from build123d import *

# Parameters (mm, degrees)
SKETCH_1_R          = 70
SKETCH_1_R_2        = 68.5
EXTRUDE_1_DEPTH     = 8
SKETCH_2_R          = 68.5
SKETCH_2_R_2        = 64
EXTRUDE_2_DEPTH     = 3
SKETCH_3_R          = 64
SKETCH_3_R_2        = 62.5
EXTRUDE_3_DEPTH     = 100
EXTRUDE_START       = 97
SKETCH_4_R          = 62.5
EXTRUDE_4_DEPTH     = 3
SKETCH_5_W          = 10
SKETCH_5_H          = 10
CUT_EXTRUDE_1_DEPTH = 10


with BuildPart() as part:
    # 스케치1 → 보스-돌출1 (new body)
    with BuildSketch(Plane(origin=(0, 0, 0), x_dir=(1, 0, 0), z_dir=(0, 1, 0))):
        with Locations(Location((0, 0, 0), (0, 0, 270))):
            Circle(SKETCH_1_R)
        with Locations(Location((0, 0, 0), (0, 0, 270))):
            Circle(SKETCH_1_R_2, mode=Mode.SUBTRACT)
    extrude(amount=EXTRUDE_1_DEPTH)

    # 스케치2 → 보스-돌출2 (add)
    with BuildSketch(Plane(origin=(0, 0, 0), x_dir=(1, 0, 0), z_dir=(0, 1, 0))):
        with Locations(Location((0, 0, 0), (0, 0, 270))):
            Circle(SKETCH_2_R)
        with Locations(Location((0, 0, 0), (0, 0, 270))):
            Circle(SKETCH_2_R_2, mode=Mode.SUBTRACT)
    extrude(amount=EXTRUDE_2_DEPTH)

    # 스케치3 → 보스-돌출3 (add)
    with BuildSketch(Plane(origin=(0, 0, 0), x_dir=(1, 0, 0), z_dir=(0, 1, 0))):
        with Locations(Location((0, 0, 0), (0, 0, 270))):
            Circle(SKETCH_3_R)
        with Locations(Location((0, 0, 0), (0, 0, 270))):
            Circle(SKETCH_3_R_2, mode=Mode.SUBTRACT)
    extrude(amount=EXTRUDE_3_DEPTH)

    # 스케치4 → 보스-돌출4 (add)
    with BuildSketch(Plane(origin=(0, 0, 0), x_dir=(1, 0, 0), z_dir=(0, 1, 0)).offset(EXTRUDE_START)):
        with Locations(Location((0, 0, 0), (0, 0, 270))):
            Circle(SKETCH_4_R)
    extrude(amount=EXTRUDE_4_DEPTH)

    # 스케치5 → 컷-돌출1 (cut)
    with BuildSketch(Plane(origin=(0, 100, 0), x_dir=(1, 0, 0), z_dir=(0, 1, 0))):
        Rectangle(SKETCH_5_W, SKETCH_5_H)
    extrude(amount=-CUT_EXTRUDE_1_DEPTH, mode=Mode.SUBTRACT)


solid = part.part
Verification items for the finished model (mm, model axes). A direction names the side the tool comes from. Coordinates: 2 decimals unless noted, no trailing zeros. Write each loop counter-clockwise with the first axis right and the second up, starting at its lowest first coordinate (ties: lowest second). Pieces come first, ordered by that corner, then holes. Notation, with made-up numbers: (50, -22.75) - (101, -22.75) arc R26 cw to (101, 7.25) - close; hole circle Ø11 at (7.25, -35). An arc over 180 degrees is marked (long way). Answer as a JSON object with one key per item and string values.
(1) Tool access check on faces 1 (the cylindrical face through (-62.48, 50.82, -13.87)), 2 (the flat face through (-13, 100, -1)), 3 (the flat face through (-13, 97, -1)). Record the directions out of +Z, -Z, +X, -X, +Y, -Y that give a thin tool (end or side, any length) a straight path to the whole face; none if there is none.
Report:
{"face 1": "+Y", "face 2": "+Z, -Z, +X, -X, +Y", "face 3": "-Y"}
(2) Cross-section at A-A on x = 0. Record the cut outline in (y, z), plus the area to 3 significant figures.
Report:
{"outline": "(0, -70) - (8, -70) - (8, -68.5) - (3, -68.5) - (3, -64) - (100, -64) - (100, -5) - (97, -5) - (97, -62.5) - (0, -62.5) - close; (0, 62.5) - (97, 62.5) - (97, 5) - (100, 5) - (100, 64) - (3, 64) - (3, 68.5) - (8, 68.5) - (8, 70) - (0, 70) - close", "area": "696 mm^2"}
(3) Mould release check, pull along Z, two halves, no side actions. Record for faces 4 (the cylindrical face through (-41.68, 5.46, -54.36)), 5 (the flat face through (-52, 8, 46)), 6 (the cylindrical face through (-42.594, 3.944, -55.55)): pulls with the +Z half, pulls with the -Z half, needs draft (parallel to the pull), parting line crosses it, or undercut.
Report:
{"face 4": "undercut", "face 5": "needs draft", "face 6": "parting line crosses it"}
(4) Cross-section at C-C on y = 45. Record the cut outline in (x, z), plus the area to 3 significant figures.
Report:
{"outline": "circle Ø128 at (0, 0); hole circle Ø125 at (0, 0)", "area": "596 mm^2"}
(5) Thickness scan on line 1 along X through (y, z) = (4.95, 0); line 2 along Z through (x, y) = (-0.5, 93.5). Record the ranges inside material, lowest first.
Report:
{"line 1": "-70 to -68.5, -64 to -62.5, 62.5 to 64, 68.5 to 70", "line 2": "-64 to -62.5, 62.5 to 64"}
(6) Cross-section at D-D on z = 59. Record the cut outline in (x, y), plus the area to 3 significant figures.
Report:
{"outline": "(-37.67, 0) - (-20.62, 0) - (-20.62, 97) - (20.62, 97) - (20.62, 0) - (37.67, 0) - (37.67, 8) - (34.8, 8) - (34.8, 3) - (24.8, 3) - (24.8, 100) - (-24.8, 100) - (-24.8, 3) - (-34.8, 3) - (-34.8, 8) - (-37.67, 8) - close", "area": "1,070 mm^2"}
(7) Gauge pin test, flat ends, axial feed: pin 1 Ø3 at (y, z) = (79.5, -10) entering from -X; pin 2 Ø3 at (x, z) = (39, 36) entering from -Y; pin 3 Ø1.5 at (x, y) = (2, 99) entering from +Z. Record the tip position at first contact, or that the pin passes through.
Report:
{"pin 1": "x = -63.43", "pin 2": "y = 97", "pin 3": "z = 63.99"}
(8) Cross-section at B-B on z = 0. Record the cut outline in (x, y).
Report:
{"outline": "(-70, 0) - (-62.5, 0) - (-62.5, 97) - (-5, 97) - (-5, 100) - (-64, 100) - (-64, 3) - (-68.5, 3) - (-68.5, 8) - (-70, 8) - close; (5, 97) - (62.5, 97) - (62.5, 0) - (70, 0) - (70, 8) - (68.5, 8) - (68.5, 3) - (64, 3) - (64, 100) - (5, 100) - close"}
